Geometry: final body of the model. Coordinates: model frame, mm. A direction names the side the tool comes from. Round coordinates to 2 decimals unless told otherwise and drop trailing zeros. Loops run counter-clockwise (first coordinate to the right, second up) from the corner with the lowest first, then second, coordinate; pieces in that order, holes last. Notation, with made-up numbers: M -27,38 L 22,38 A19 ccw 22,67 Z; hole C 11,2.25 d4. An arc over 180 degrees is marked long. Write each question's results on one line, items separated by ' | '.
```python
from build123d import *

# Parameters (mm, degrees)
ESQUISSE1_W        = 21
ESQUISSE1_H        = 41
ESQUISSE1_R        = 0.75
ESQUISSE1_R_2      = 2
ESQUISSE1_R_3      = 3
BOSS_EXTRU_1_DEPTH = 2
BOSS_EXTRU_2_START = 2
ESQUISSE1_3_R      = 0.75
ESQUISSE1_3_R_2    = 3
BOSS_EXTRU_2_DEPTH = 8


with BuildPart() as part:
    # Esquisse1 → Boss.-Extru.1 (new body)
    with BuildSketch(Plane.XY):
        with BuildLine():
            Line((-15, 100), (-15, 50))
            ThreePointArc((-15, 50), (-15.138914933, 48.338975829), (-15.551800259, 46.72409987))
            Line((-15.551800259, 46.72409987), (-28.344599222, 9.827700389))
            ThreePointArc((-28.344599222, 9.827700389), (0, -30), (28.344599222, 9.827700389))
            Line((28.344599222, 9.827700389), (15.551800259, 46.72409987))
            ThreePointArc((15.551800259, 46.72409987), (15.138914933, 48.338975829), (15, 50))
            Line((15, 50), (15, 100))
            ThreePointArc((15, 100), (0, 115), (-15, 100))
        make_face()
        with Locations((-0.323225061, 82.579304785)):
            Rectangle(ESQUISSE1_W, ESQUISSE1_H, mode=Mode.SUBTRACT)
        with Locations((0, -7.5)):
            Circle(ESQUISSE1_R, mode=Mode.SUBTRACT)
        with Locations((-7.5, 0)):
            Circle(ESQUISSE1_R, mode=Mode.SUBTRACT)
        with Locations((0, 7.5)):
            Circle(ESQUISSE1_R, mode=Mode.SUBTRACT)
        with Locations((7.5, 0)):
            Circle(ESQUISSE1_R, mode=Mode.SUBTRACT)
        with Locations((4.676774939, 106.958577425)):
            Circle(ESQUISSE1_R_2, mode=Mode.SUBTRACT)
        with Locations((-5.323225061, 106.958577425)):
            Circle(ESQUISSE1_R_2, mode=Mode.SUBTRACT)
        with Locations((4.676774939, 58.328577425)):
            Circle(ESQUISSE1_R_2, mode=Mode.SUBTRACT)
        with Locations((-5.323225061, 58.328577425)):
            Circle(ESQUISSE1_R_2, mode=Mode.SUBTRACT)
        Circle(ESQUISSE1_R_3, mode=Mode.SUBTRACT)
    extrude(amount=BOSS_EXTRU_1_DEPTH)

    # Esquisse1<3> → Boss.-Extru.2 (add)
    with BuildSketch(Plane.XY.offset(BOSS_EXTRU_2_START)):
        with BuildLine():
            ThreePointArc((-10.823225061, 110.385460957), (-13.916687392, 105.596946672), (-15, 100))
            Line((-15, 100), (-15, 50))
            ThreePointArc((-15, 50), (-15.138914933, 48.338975829), (-15.551800259, 46.72409987))
            Line((-15.551800259, 46.72409987), (-28.344599222, 9.827700389))
            ThreePointArc((-28.344599222, 9.827700389), (0, -30), (28.344599222, 9.827700389))
            Line((28.344599222, 9.827700389), (15.551800259, 46.72409987))
            ThreePointArc((15.551800259, 46.72409987), (15.138914933, 48.338975829), (15, 50))
            Line((15, 50), (15, 100))
            ThreePointArc((15, 100), (13.74139047, 106.014498147), (10.176774939, 111.019675668))
            Line((10.176774939, 111.019675668), (10.176774939, 55.229304785))
            Line((10.176774939, 55.229304785), (-10.823225061, 55.229304785))
            Line((-10.823225061, 55.229304785), (-10.823225061, 110.385460957))
        make_face()
        with Locations((0, -7.5)):
            Circle(ESQUISSE1_3_R, mode=Mode.SUBTRACT)
        with Locations((7.5, 0)):
            Circle(ESQUISSE1_3_R, mode=Mode.SUBTRACT)
        with Locations((0, 7.5)):
            Circle(ESQUISSE1_3_R, mode=Mode.SUBTRACT)
        with Locations((-7.5, 0)):
            Circle(ESQUISSE1_3_R, mode=Mode.SUBTRACT)
        Circle(ESQUISSE1_3_R_2, mode=Mode.SUBTRACT)
    extrude(amount=BOSS_EXTRU_2_DEPTH)


solid = part.part
```
1. Section B-B (y = 83.5). Output: boundary loops of the cut face in (x, z), then the cut area to 3 significant figures.
Answer key:
outline: M -15,0 L -10.82,0 L -10.82,10 L -15,10 Z; M 10.18,0 L 15,0 L 15,10 L 10.18,10 Z | area: 90.0 mm²
2. Section A-A (z = 6.75). Output: boundary loops of the cut face in (x, y), then the cut area to 3 significant figures.
Answer key:
outline: M -28.34,9.83 A30 ccw long 28.34,9.83 L 15.55,46.72 A10 cw 15,50 L 15,100 A15 ccw 10.18,111.02 L 10.18,55.23 L -10.82,55.23 L -10.82,110.39 A15 ccw -15,100 L -15,50 A10 cw -15.55,46.72 Z; hole C -7.5,0 d1.5; hole C 0,0 d6; hole C 0,-7.5 d1.5; hole C 0,7.5 d1.5; hole C 7.5,0 d1.5 | area: 4,300 mm²
3. Ray query, probe 1 along X at (y, z) = (58, 1); probe 2 along Y at (x, z) = (0, 3.25); probe 3 along X at (y, z) = (74.5, 5). Return the intervals inside material, ascending.
Answer key:
probe 1: x = -15 to -7.3, -3.35 to 2.7, 6.65 to 15 | probe 2: y = -30 to -8.25, -6.75 to -3, 3 to 6.75, 8.25 to 55.23 | probe 3: x = -15 to -10.82, 10.18 to 15
4. Draft query along Y for faces 4 (the face through (-0.8, -29.99, 4.93)), 5 (the face through (-15, 75, 5)), 6 (the face through (-10.823, 82, 5)). Return one class per face: pulls with the +Y half, pulls with the -Y half, needs draft (parallel to the pull), parting line crosses it, or undercut.
Answer key:
face 4: parting line crosses it | face 5: needs draft | face 6: undercut
5. Pin query (flat end, axial travel): P1, Ø3, axis at x = -8.5, z = 8.5, coming from the +Y side; P2, Ø3.5, axis at x = -3, y = 59.5, coming from the +Z side; P3, Ø3, axis at y = 95, z = 3.5, coming from the -X side. Return the tip coordinate at first contact, or that it passes through.
Answer key:
P1: stops at y = 55.23 | P2: stops at z = 2 | P3: stops at x = -15
6. Access query for faces 1 (the face through (-5.584, 108.942, 0.986)), 2 (the face through (0, 55.229, 6)), 3 (the face through (15, 75, 5)). Directions: +Z, -Z, +X, -X, +Y, -Y. A direction counts if a zero-diameter tool reaches every point of the face in a straight line with its end or side. Return the directions, or none.
Answer key:
face 1: +Z, -Z | face 2: +Z, +Y | face 3: +Z, -Z, +X, +Y
7. Section C-C (x = 19). Output: boundary loops of the cut face in (y, z), then the cut area to 3 significant figures.
Answer key:
outline: M -23.22,0 L 36.78,0 L 36.78,10 L -23.22,10 Z | area: 600 mm²
8. Section D-D (y = -17.5). Output: boundary loops of the cut face in (x, z).
Answer key:
outline: M -24.37,0 L 24.37,0 L 24.37,10 L -24.37,10 Z
